Here's how the part is built. I have some questions about the finished solid (model axes, mm). Face numbers are marked on the shaded views. A direction names the side the tool comes from. Round coordinates to 2 decimals unless told otherwise and drop trailing zeros. Write each loop counter-clockwise with the first axis right and the second up, starting at its lowest first coordinate (ties: lowest second). Pieces come first, ordered by that corner, then holes. Notation, with made-up numbers: (66.5, -35.5) -> (116.5, -35.5) arc R36 cw to (116.5, -0.5) -> close; hole circle Ø8 at (6, -27.5). An arc over 180 degrees is marked (long way). Answer as CSV lines item,"result".
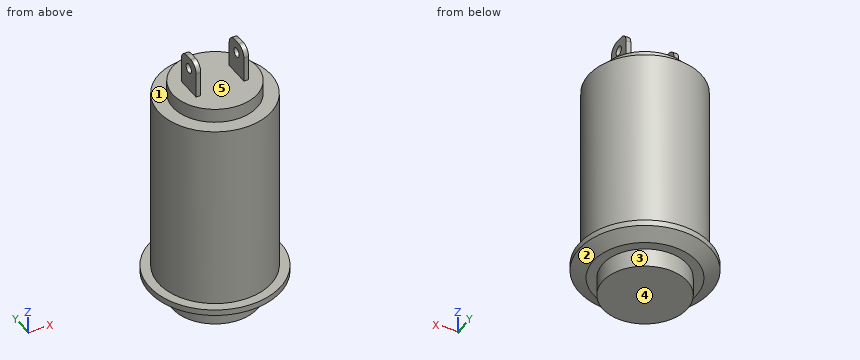
from build123d import *

# Parameters (mm, degrees)
SKETCH_1_R          = 4.5
EXTRUDE_1_DEPTH     = 2
SKETCH_2_R          = 7
EXTRUDE_2_DEPTH     = 1.5
SKETCH_3_R          = 6
EXTRUDE_3_DEPTH     = 20
SKETCH_4_R          = 4.5
EXTRUDE_4_DEPTH     = 1.5
SKETCH_5_W          = 0.5
SKETCH_5_H          = 2.8
EXTRUDE_5_DEPTH     = 3.7
CHAMFER_1_SIZE      = 1.5
CHAMFER_1_SIZE2     = 0.866025404
FILLET_1_R          = 1
SKETCH_6_R          = 0.5
CUT_EXTRUDE_1_DEPTH = 32.124427706


with BuildPart() as part:
    # 스케치1 → 보스-돌출1 (new body)
    with BuildSketch(Plane.XY):
        Circle(SKETCH_1_R)
    extrude(amount=EXTRUDE_1_DEPTH)

    # 스케치2 → 보스-돌출2 (add)
    with BuildSketch(Plane.XY.offset(2)):
        Circle(SKETCH_2_R)
    extrude(amount=EXTRUDE_2_DEPTH)

    # 스케치3 → 보스-돌출3 (add)
    with BuildSketch(Plane.XY.offset(3.5)):
        Circle(SKETCH_3_R)
    extrude(amount=EXTRUDE_3_DEPTH)

    # 스케치4 → 보스-돌출4 (add)
    with BuildSketch(Plane.XY.offset(23.5)):
        Circle(SKETCH_4_R)
    extrude(amount=EXTRUDE_4_DEPTH)

    # 스케치5 → 보스-돌출5 (add)
    with BuildSketch(Plane.XY.offset(25)):
        with Locations((2.55, 0)):
            Rectangle(SKETCH_5_W, SKETCH_5_H)
        with Locations((-2.55, 0)):
            Rectangle(SKETCH_5_W, SKETCH_5_H)
    extrude(amount=EXTRUDE_5_DEPTH)

    # 모따기1
    chamfer_1_edges = [part.edges().sort_by_distance(p)[0] for p in [
        (-7, 0, 2),
    ]]
    chamfer_1_side = [part.faces().sort_by_distance(p)[0] for p in [
        (-6.802010101, 0, 2),
    ]]
    chamfer(chamfer_1_edges, length=CHAMFER_1_SIZE, length2=CHAMFER_1_SIZE2, reference=chamfer_1_side[0])

    # 필렛1
    fillet_1_edges = [part.edges().sort_by_distance(p)[0] for p in [
        (-2.55, 1.4, 28.7),
        (-2.55, -1.4, 28.7),
        (2.55, 1.4, 28.7),
        (2.55, -1.4, 28.7),
    ]]
    fillet(fillet_1_edges, radius=FILLET_1_R)

    # 스케치6 → 컷-돌출1 (cut, through all)
    with BuildSketch(Plane.ZY.offset(2.8)):
        with Locations((27.421769494, 0)):
            Circle(SKETCH_6_R)
    extrude(amount=-CUT_EXTRUDE_1_DEPTH, mode=Mode.SUBTRACT)


solid = part.part
Item 1: Suppose I cut it at C-C, the plane z = 4.5. List the corners of the cut face in (x, y) for me.
Results found:
outline,"circle Ø12 at (0, 0)"
Item 2: Will these pins go through, and if not, where does the flat tip stop? pin 1 (2 mm diameter, centred on y = 0.5, z = 27, fed in from +X); pin 2 (6 mm diameter, centred on x = -5.5, y = 4.5, fed in from +Z); pin 3 (3 mm diameter, centred on x = 0, z = 19.5, fed in from +Y).
Results found:
pin 1,"stops at x = 2.8"
pin 2,"stops at z = 25"
pin 3,"stops at y = 6"
Item 3: I need wall thicknesses on L1, parallel to X at y = -1, z = 25.5; L2, parallel to Z at x = 2.75, y = 3.75; L3, parallel to Z at x = -3.25, y = -2.75. Which ranges of each line are inside material? Lowest first, please.
Results found:
L1,"x = -2.8 to -2.3, 2.3 to 2.8"
L2,"z = 2 to 23.5"
L3,"z = 0 to 25"
Item 4: Suppose I cut it at A-A, the plane y = 0. State how many separate pieces and enclosed holes the cut face has, then the cut area to 3 significant figures.
Results found:
separate pieces,"3"
enclosed holes,"0"
area,"294 mm²"
Item 5: If we mould it in two halves opening along X, with no side actions, what happens to the marked faces 3, 4 and 5? For each: pulls with the +X half, pulls with the -X half, needs draft (parallel to the pull), parting line crosses it, or undercut.
Results found:
face 3,"parting line crosses it"
face 4,"needs draft"
face 5,"undercut"
Item 6: For the marked faces 1 and 2, which set-ups out of +Z, -Z, +X, -X, +Y, -Y let a thin tool reach every point of the face, with its end or its side?
Results found:
face 1,"+Z"
face 2,"-Z"
Item 7: Suppose I cut it at B-B, the plane x = 0. List the corners of the cut face in (y, z) for me, then the cut area to 3 significant figures.
Results found:
outline,"(-7, 2.87) -> (-5.5, 2) -> (-4.5, 2) -> (-4.5, 0) -> (4.5, 0) -> (4.5, 2) -> (5.5, 2) -> (7, 2.87) -> (7, 3.5) -> (6, 3.5) -> (6, 23.5) -> (4.5, 23.5) -> (4.5, 25) -> (-4.5, 25) -> (-4.5, 23.5) -> (-6, 23.5) -> (-6, 3.5) -> (-7, 3.5) -> close"
area,"291 mm²"
